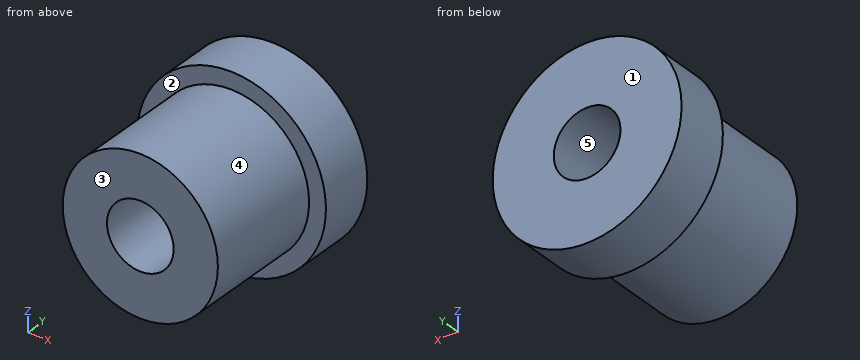
```python
from build123d import *

# Parameters (mm, degrees)
SKETCH1_R           = 5.55625
BASE_EXTRUDE_DEPTH  = 12.7
SKETCH2_R           = 6.76275
BOSS_EXTRUDE1_DEPTH = 3.9624
SKETCH3_R           = 2.3876
CUT_EXTRUDE1_DEPTH  = 16.898414233


with BuildPart() as part:
    # Sketch1 → Base-Extrude (new body)
    with BuildSketch(Plane(origin=(0, 0, 0), x_dir=(1, 0, 0), z_dir=(0, 1, 0))):
        with Locations(Location((0, 0, 0), (0, 0, 270))):
            Circle(SKETCH1_R)
    extrude(amount=-BASE_EXTRUDE_DEPTH)

    # Sketch2 → Boss-Extrude1 (add)
    with BuildSketch(Plane(origin=(0, 0, 0), x_dir=(-1, 0, 0), z_dir=(0, 1, 0))):
        with Locations(Location((0, 0, 0), (0, 0, 90))):
            Circle(SKETCH2_R)
    extrude(amount=-BOSS_EXTRUDE1_DEPTH)

    # Sketch3 → Cut-Extrude1 (cut, through all)
    with BuildSketch(Plane(origin=(0, 0, 0), x_dir=(-1, 0, 0), z_dir=(0, 1, 0))):
        with Locations(Location((0, 0, 0), (0, 0, 90))):
            Circle(SKETCH3_R)
    extrude(amount=-CUT_EXTRUDE1_DEPTH, mode=Mode.SUBTRACT)


solid = part.part
```
Build history of the part. All positions in model axes, mm. Face numbers are marked on the shaded views. A direction names the side the tool comes from. Coordinates: 2 decimals unless noted, no trailing zeros. Write each loop counter-clockwise with the first axis right and the second up, starting at its lowest first coordinate (ties: lowest second). Pieces come first, ordered by that corner, then holes.
1. Band-saw the part on D-D, the plane x = -3. Give the cut face in (y, z).
Answer block:
outline: (-12.7, -4.68) - (-3.96, -4.68) - (-3.96, -6.06) - (0, -6.06) - (0, 6.06) - (-3.96, 6.06) - (-3.96, 4.68) - (-12.7, 4.68) - close
2. 3-axis set-ups, long thin cutter, end or side, ignore diameter. For the marked faces 1 and 2: which of +Z, -Z, +X, -X, +Y, -Y reach the whole face in a straight line?
Answer block:
face 1: +Z, -Z, +X, -X, +Y
face 2: -Y
3. Drop flat-ended pins along their axis: pin 1 (1.5 mm diameter, centred on y = -6, z = -3.5, fed in from +X); pin 2 (5 mm diameter, centred on x = -5, y = -9, fed in from +Z); pin 3 (2 mm diameter, centred on y = -10, z = -0.5, fed in from -X). Give the stop position or say it passes through.
Answer block:
pin 1: stops at x = 4.83
pin 2: stops at z = 4.96
pin 3: stops at x = -5.56
4. Drill centre lines: probe 1 along X at (y, z) = (-5.25, 0); probe 2 along X at (y, z) = (-2.5, 0); probe 3 along Y at (x, z) = (-5.75, -2.75). Where is each one in solid material? Low to high.
Answer block:
probe 1: x = -5.56 to -2.39, 2.39 to 5.56
probe 2: x = -6.76 to -2.39, 2.39 to 6.76
probe 3: y = -3.96 to 0
5. Pull direction X, two halves, no side cores. Call the marked faces 3, 4 and 5: released by +X, released by -X, zero draft, split by the parting line, or undercut.
Answer block:
face 3: zero draft
face 4: split by the parting line
face 5: undercut
6. Band-saw the part on A-A, the plane z = 0. Give the cut face in (x, y).
Answer block:
outline: (-6.76, -3.96) - (-5.56, -3.96) - (-5.56, -12.7) - (-2.39, -12.7) - (-2.39, 0) - (-6.76, 0) - close; (2.39, -12.7) - (5.56, -12.7) - (5.56, -3.96) - (6.76, -3.96) - (6.76, 0) - (2.39, 0) - close
7. Band-saw the part on B-B, the plane x = 0. Give the cut face in (y, z), and give its area (3 significant figures).
Answer block:
outline: (-12.7, -5.56) - (-3.96, -5.56) - (-3.96, -6.76) - (0, -6.76) - (0, -2.39) - (-12.7, -2.39) - close; (-12.7, 2.39) - (0, 2.39) - (0, 6.76) - (-3.96, 6.76) - (-3.96, 5.56) - (-12.7, 5.56) - close
area: 90.0 mm2
8. Band-saw the part on C-C, the plane y = -8.75. Give the cut face in (x, z).
Answer block:
outline: circle Ø11.11 at (0, 0); hole circle Ø4.78 at (0, 0)
